Can you work these out from the model? Positions are in its coordinate system, mm. Face numbers are marked on the shaded views. A direction names the side the tool comes from. Give positions to 0.01 mm unless a question says otherwise; leave off trailing zeros. Loops run counter-clockwise (first coordinate to the right, second up) from the corner with the lowest first, then second, coordinate; pieces in that order, holes last. Notation, with made-up numbers: (16.5, -37.75) - (23.5, -37.75) arc R23 ccw to (23.5, -20.75) - close; hole circle Ø8 at (57, -22.75). An arc over 180 degrees is marked (long way). Write item = value, one per line.
from build123d import *

# Parameters (mm, degrees)
SKETCH1_W                 = 44.45
SKETCH1_H                 = 25.908
BOSS_EXTRUDE1_DEPTH       = 30.48
SIDECHAMFER_SIZE          = 12.7
BACKCHAMFERS_SIZE         = 6.35
SKETCH2_W                 = 12.065
SKETCH2_H                 = 11.938
LINACTSLOT_DEPTH          = 46.762489978
MOUTINGHOLES_D            = 2.7051
MOUTINGHOLES_DEPTH        = 14.478
MOUTINGHOLES_TIP          = 0.81269403
CUT_EXTRUDE1_DEPTH        = 46.762489978
MOTORMOUNTINGHOLES2_D     = 2.2606
MOTORMOUNTINGHOLES2_DEPTH = 11.43
MOTORMOUNTINGHOLES2_TIP   = 0.679152758
GRIPPERSETSCREW_D         = 2.2606


with BuildPart() as part:
    # Sketch1 → Boss-Extrude1 (new body)
    with BuildSketch(Plane(origin=(0, 0, 0), x_dir=(1, 0, 0), z_dir=(0, 1, 0))):
        Rectangle(SKETCH1_W, SKETCH1_H)
    extrude(amount=BOSS_EXTRUDE1_DEPTH)

    # SideChamfer
    sidechamfer_edges = [part.edges().sort_by_distance(p)[0] for p in [
        (22.225, 0, 0),
    ]]
    chamfer(sidechamfer_edges, length=SIDECHAMFER_SIZE)

    # BackChamfers
    backchamfers_edges = [part.edges().sort_by_distance(p)[0] for p in [
        (22.225, 21.59, 12.954),
        (-22.225, 15.24, 12.954),
    ]]
    chamfer(backchamfers_edges, length=BACKCHAMFERS_SIZE)

    # Sketch2 → LinActSlot (cut, through all)
    with BuildSketch(Plane.XY.offset(12.954)):
        with Locations((0, 24.511)):
            Rectangle(SKETCH2_W, SKETCH2_H)
    extrude(amount=-LINACTSLOT_DEPTH, mode=Mode.SUBTRACT)

    # MoutingHoles
    with Locations(Plane(origin=(14.160350453, 30.48, 8.373414988), x_dir=(-1, 0, 0), z_dir=(0, 1, 0))):
        with Locations((1.460350453, -4.309414988), (26.860350453, -4.309414988)):
            Hole(MOUTINGHOLES_D / 2, depth=MOUTINGHOLES_DEPTH)
            with Locations((0, 0, -(MOUTINGHOLES_DEPTH + MOUTINGHOLES_TIP / 2))):  # 118° drill point
                Cone(0, MOUTINGHOLES_D / 2, MOUTINGHOLES_TIP, mode=Mode.SUBTRACT)

    # Sketch11 → Cut-Extrude1 (cut, through all)
    with BuildSketch(Plane(origin=(0, 0, -12.954), x_dir=(-1, 0, 0), z_dir=(0, 0, -1))):
        with BuildLine():
            Line((16.51, 6.35), (16.51, 0))
            Line((16.51, 0), (-3.81, 0))
            Line((-3.81, 0), (-3.81, 6.35))
            ThreePointArc((-3.81, 6.35), (6.35, 16.51), (16.51, 6.35))
        make_face()
    extrude(amount=-CUT_EXTRUDE1_DEPTH, mode=Mode.SUBTRACT)

    # MotorMountingHoles2
    with Locations(Plane(origin=(0, 0, -12.954), x_dir=(-1, 0, 0), z_dir=(0, 0, -1))):
        with Locations((18.8468, 6.35), (-6.1468, 6.35)):
            Hole(MOTORMOUNTINGHOLES2_D / 2, depth=MOTORMOUNTINGHOLES2_DEPTH)
            with Locations((0, 0, -(MOTORMOUNTINGHOLES2_DEPTH + MOTORMOUNTINGHOLES2_TIP / 2))):  # 118° drill point
                Cone(0, MOTORMOUNTINGHOLES2_D / 2, MOTORMOUNTINGHOLES2_TIP, mode=Mode.SUBTRACT)

    # GripperSetScrew (through all)
    with Locations(Plane(origin=(0, 18.542, 0), x_dir=(1, 0, 0), z_dir=(0, 1, 0))):
        with Locations((0, -6.604)):
            Hole(GRIPPERSETSCREW_D / 2)


solid = part.part
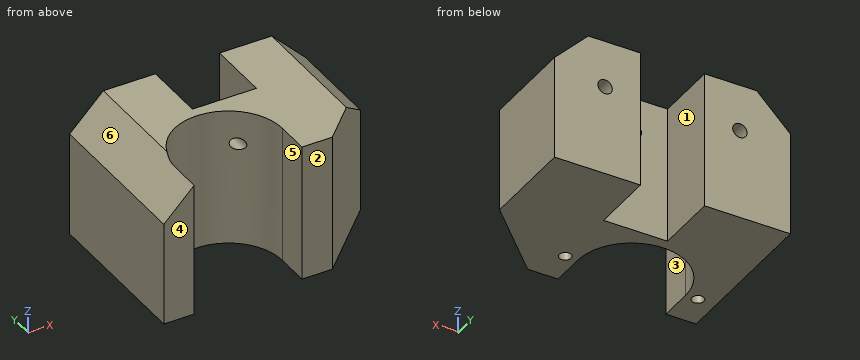
Q1. Imagine slicing it at C-C, the plane z = -7. Give the number of separate pieces and of enclosed holes in the cut face, then the cut area to 3 significant figures.
Output:
separate_pieces = 1
enclosed_holes = 2
area = 831 mm2
Q2. We'd pull the mould along X, two halves only. Please class the marked faces 4, 5 and 6: released by +X, released by -X, zero draft, split by the parting line, or undercut.
Output:
face_4 = zero draft
face_5 = undercut
face_6 = released by -X
Q3. Imagine slicing it at D-D, the plane x = 2.5. Write out the boundary of the cut face in (y, z), then the cut area to 3 significant figures.
Output:
outline = (11.34, -12.95) - (18.54, -12.95) - (18.54, 12.95) - (11.34, 12.95) - close
area = 187 mm2
Q4. Imagine slicing it at A-A, the plane y = 14.5. Write out the boundary of the cut face in (x, z) (3 decimals), then the cut area to 3 significant figures.
Output:
outline = (-22.225, -12.954) - (-12.417, -12.954) - (-12.417, 12.954) - (-15.875, 12.954) - (-22.225, 6.604) - close; (-0.283, -12.954) - (22.225, -12.954) - (22.225, 6.604) - (15.875, 12.954) - (-0.283, 12.954) - (-0.283, 7.698) arc R1.13 cw (long way) to (-0.283, 5.51) - close
area = 794 mm2
Q5. For pin 1 (1.9 mm diameter, centred on y = 4, z = -2, fed in from +X) (3 decimals); pin 2 (8 mm diameter, centred on x = 1, z = -10.5, fed in from +Y); pin 3 (1.4 mm diameter, centred on x = 6.15, y = 6.35, fed in from -Z); pin 4 (1.8 mm diameter, centred on x = 0, z = 6.604, fed in from +Y), each with a flat end and sliding along its axis, tell me the tip position at first contact or that it passes through.
Output:
pin_1 = 14.475
pin_2 = 18.54
pin_3 = -1.27
pin_4 = through
Q6. I need wall thicknesses on L1, parallel to X at y = 26.5, z = -10 (1 decimal); L2, parallel to Z at x = 0, y = 16.95; L3, parallel to X at y = 3, z = 6 (3 decimals). Which ranges of each line are inside material? Lowest first, please.
Output:
L1 = -22.2 to -6, 6 to 22.2
L2 = -12.95 to 5.47, 7.73 to 12.95
L3 = -22.225 to -16.51, 3.81 to 12.525
Q7. Which directions (+Z, -Z, +X, -X, +Y, -Y) give clear straight access to the entire face, cutting with the end or side of a thin tool? Please do the marked faces 1, 2 and 3.
Output:
face_1 = +Z, -Z, +Y
face_2 = +Z, -Z, +X, -X, -Y
face_3 = +Z, -Z, -Y
